Source: CAD feature listing. Evaluate the final solid. Frame: model axes, mm. A direction names the side the tool comes from. Round coordinates to 2 decimals unless told otherwise and drop trailing zeros. Loops run counter-clockwise (first coordinate to the right, second up) from the corner with the lowest first, then second, coordinate; pieces in that order, holes last. Notation, with made-up numbers: M -35,-13 L -18,-13 A17 ccw -18,-6 Z; hole C 19,-6 d8. An arc over 180 degrees is marked long. One line per item, written item: value.
from build123d import *

# Parameters (mm, degrees)
F1_DEPTH = 31.75
F2_W     = 111.76
F2_H     = 60.96
F3_DEPTH = 19.05
F4_R     = 1.397
F5_DEPTH = 127.001
F6_R     = 1.397
F7_DEPTH = 76.201


with BuildPart() as f1:
    # F0 (on Top) → F1 (new body)
    with BuildSketch(Plane.XY):
        Polygon((63.5, 0), (0, 0), (-63.5, 0), (-63.5, -76.2), (63.5, -76.2), align=None)
    extrude(amount=F1_DEPTH)

    # F2 (on face) → F3 (cut)
    with BuildSketch(Plane.XY.offset(31.75)):
        with Locations((0, -38.1)):
            Rectangle(F2_W, F2_H)
    extrude(amount=-F3_DEPTH, mode=Mode.SUBTRACT)

    # F4 (on face) → F5 (cut, through all)
    with BuildSketch(Plane.YZ.offset(63.5)):
        with Locations((-38.1, 15.875)):
            Circle(F4_R)
    extrude(amount=-F5_DEPTH, mode=Mode.SUBTRACT)

    # F6 (on face) → F7 (cut, through all)
    with BuildSketch(Plane.XZ.offset(76.2)):
        with Locations((0, 15.875)):
            Circle(F6_R)
    extrude(amount=-F7_DEPTH, mode=Mode.SUBTRACT)


solid = f1.part
1. Section query C-C (y = -38.1). Return the cut outline in (x, z), and give its area (3 significant figures).
Report:
outline: M -63.5,0 L 63.5,0 L 63.5,14.48 L 55.88,14.48 L 55.88,12.7 L -55.88,12.7 L -55.88,14.48 L -63.5,14.48 Z; M -63.5,17.27 L -55.88,17.27 L -55.88,31.75 L -63.5,31.75 Z; M 55.88,17.27 L 63.5,17.27 L 63.5,31.75 L 55.88,31.75 Z
area: 1,860 mm2
2. Ray query, line 1 (Z direction, x = 0, y = -73); line 2 (Y direction, x = -19.5, z = 29); line 3 (X direction, y = -60, z = 21.5). Return the intervals inside material, ascending. Write a range as [from, to].
Report:
line 1: z = [0, 14.48], [17.27, 31.75]
line 2: y = [-76.2, -68.58], [-7.62, 0]
line 3: x = [-63.5, -55.88], [55.88, 63.5]
3. Section query D-D (y = -13). Return the cut outline in (x, z).
Report:
outline: M -63.5,0 L 63.5,0 L 63.5,31.75 L 55.88,31.75 L 55.88,12.7 L -55.88,12.7 L -55.88,31.75 L -63.5,31.75 Z
4. Section query A-A (x = 0). Return the cut outline in (y, z).
Report:
outline: M -76.2,0 L 0,0 L 0,14.48 L -7.62,14.48 L -7.62,12.7 L -68.58,12.7 L -68.58,14.48 L -76.2,14.48 Z; M -76.2,17.27 L -68.58,17.27 L -68.58,31.75 L -76.2,31.75 Z; M -7.62,17.27 L 0,17.27 L 0,31.75 L -7.62,31.75 Z
5. Pin query (flat end, axial travel): pin 1 (3.5 mm diameter, centred on x = 0, z = 15.875, fed in from -Y). Return the tip coordinate at first contact, or that it passes through.
Report:
pin 1: stops at y = -76.2
6. Reachability of faces 1 (the face through (-55.88, -39, 22)), 2 (the face through (63.5, -39, 12)) from +Z, -Z, +X, -X, +Y, -Y: full face, straight path, thin tool, end or side. Return the list, or none.
Report:
face 1: +Z
face 2: +Z, -Z, +X, +Y, -Y
7. Section query B-B (z = 23.5). Return the cut outline in (x, y).
Report:
outline: M -63.5,-76.2 L 63.5,-76.2 L 63.5,0 L -63.5,0 Z; hole M -55.88,-68.58 L 55.88,-68.58 L 55.88,-7.62 L -55.88,-7.62 Z
8. Pull-direction query (Y, two-part tool) for faces 3 (the face through (-1, -38, 12.7)), 4 (the face through (-0.18, -72.44, 17.26)), 5 (the face through (-1, -76.2, 12)); classes: released by +Y, released by -Y, zero draft, split by the parting line, or undercut.
Report:
face 3: undercut
face 4: zero draft
face 5: released by -Y
